Read the model definition and answer for the solid it produces. Units are mm, in the model's axes. A direction names the side the tool comes from. Give positions to 0.01 mm unless a question says otherwise; leave off trailing zeros. Order: outer loops, then holes, each group sorted by start corner. A loop starts at its lowest first (then second) coordinate and runs counter-clockwise, first axis right, second up. Notation, with made-up numbers: (63.25, 80.25) -> (72.25, 80.25) arc R15 ccw to (72.25, 92.25) -> close; hole circle Ø1 at (56.25, 57). An arc over 180 degrees is marked (long way). Answer as CSV lines item,"result". Start each with the question number.
1) Straight lines are drawn through the part: L1, parallel to Y at x = 15.7, z = 0; L2, parallel to Y at x = 10, z = 57. For each, find the intervals that lie inside material, in ascending order. Write a range as from..to.
2) The mould has two halves that part along Y. Classify faces 3 (the face through (0, -16, -1)), 4 (the face through (15.189, -0.33, 7.493)), 5 (the face through (-1, -15, -83)): +Y half, -Y half, draft (parallel to the pull), parting line (faces both ways), or undercut.
3) Find section C-C (y = 0). Determine the outline of the cut face in (x, z), and give its area (3 significant figures).
4) Find section B-B (y = -10.5). Determine the outline of the cut face in (x, z).
5) Find section A-A (z = 0). Determine the outline of the cut face in (x, y).
6) For faces 1 (the face through (14.4, -9, -1)), 2 (the face through (16, -11, -1)), determine the directions among +Z, -Z, +X, -X, +Y, -Y from which every point of the face is accessible in a straight line to the end or side of a thin tool.
7) Flat-ended cylindrical pins translate along their axes: pin 1 Ø12 at (x, y) = (-2, -9) entering from -Z; pin 2 Ø8 at (x, y) = (11.5, 3) entering from -Z. Find the tip coordinate at first contact, or state that the pin passes through.
8) Find section D-D (x = -1.5). Determine the outline of the cut face in (y, z), and give its area (3 significant figures).
Autodesk Inventor part; units mm, degrees
ref_plane "YZ Plane" through (0, 0, 0) normal (1, 0, 0) x (0, 1, 0)
ref_plane "XZ Plane" through (0, 0, 0) normal (0, 1, 0) x (-1, 0, 0)
ref_plane "XY Plane" through (0, 0, 0) normal (0, 0, 1) x (1, 0, 0)
sketch "スケッチ1" plane through (0, 0, 0) normal (0, 0, 1) x (1, 0, 0)
  line L0 (-16, -16) -> (16, -16)
  line L1 (16, -16) -> (16, 16)
  line L2 (16, 16) -> (-16, 16)
  line L3 (-16, 16) -> (-16, -16)
  line L4 (-16, -16) -> (16, 16) construction
  line L5 (16, -16) -> (-16, 16) construction
  line L6 (-14.4, 14.4) -> (14.4, 14.4)
  line L7 (14.4, 14.4) -> (14.4, -14.4)
  line L8 (14.4, -14.4) -> (-14.4, -14.4)
  line L9 (-14.4, -14.4) -> (-14.4, 14.4)
  point P0 (0, 0)
  dimension "d0" = 32
  dimension "d1" = 32
  dimension "d2" = 1.6
extrude "押し出し1" add sketch "スケッチ1" along normal mid plane 200
chamfer "面取り1" distance 32 angle 45 1 edges at (-16, 0, 100)
chamfer "面取り2" distance 32 angle 45 1 edges at (-16, 0, -100)
sketch "スケッチ2" plane through (16, -16, 100) normal (1, 0, 0) x (0, 0, -1)
  point P0 (100, 16)
  point P1 (100, 16)
hole "穴1" at (16, 0, 0) direction (-1, 0, 0) diameter 15 end through all
properties part number "Pipe横"
Findings below:
1,L1,"-16..-7.5, 7.5..16"
1,L2,"-16..-14.4, 14.4..16"
2,face 3,"-Y half"
2,face 4,"undercut"
2,face 5,"draft"
3,outline,"(-16, -68) -> (-14.4, -69.6) -> (-14.4, -7.5) -> (-16, -7.5) -> close; (-16, 7.5) -> (-14.4, 7.5) -> (-14.4, 69.6) -> (-16, 68) -> close; (14.4, -98.4) -> (16, -100) -> (16, -7.5) -> (14.4, -7.5) -> close; (14.4, 7.5) -> (16, 7.5) -> (16, 100) -> (14.4, 98.4) -> close"
3,area,"490 mm²"
4,outline,"(-16, -68) -> (-14.4, -69.6) -> (-14.4, 69.6) -> (-16, 68) -> close; (14.4, -98.4) -> (16, -100) -> (16, 100) -> (14.4, 98.4) -> close"
5,outline,"(-16, -16) -> (16, -16) -> (16, -7.5) -> (14.4, -7.5) -> (14.4, -14.4) -> (-14.4, -14.4) -> (-14.4, -7.5) -> (-16, -7.5) -> close; (-16, 7.5) -> (-14.4, 7.5) -> (-14.4, 14.4) -> (14.4, 14.4) -> (14.4, 7.5) -> (16, 7.5) -> (16, 16) -> (-16, 16) -> close"
6,face 1,"+Z, -Z"
6,face 2,"+Z, -Z, +X, +Y, -Y"
7,pin 1,"z = -84.62"
7,pin 2,"z = -99.5"
8,outline,"(-16, -82.5) -> (-14.4, -82.5) -> (-14.4, 82.5) -> (-16, 82.5) -> close; (14.4, -82.5) -> (16, -82.5) -> (16, 82.5) -> (14.4, 82.5) -> close"
8,area,"528 mm²"
